```python
from build123d import *

# Parameters (mm, degrees)
SKETCH1_W           = 165
SKETCH1_H           = 50
BOSS_EXTRUDE1_DEPTH = 2.5
FILLET1_R           = 25
SKETCH2_R           = 2.5
CUT_EXTRUDE1_DEPTH  = 2.5
SKETCH4_R           = 2.25
BOSS_EXTRUDE2_DEPTH = 8


with BuildPart() as part:
    # Sketch1 → Boss-Extrude1 (new body)
    with BuildSketch(Plane.XY):
        Rectangle(SKETCH1_W, SKETCH1_H)
    extrude(amount=BOSS_EXTRUDE1_DEPTH)

    # Fillet1
    fillet1_edges = [part.edges().sort_by_distance(p)[0] for p in [
        (-82.5, -25, 1.25),
        (-82.5, 25, 1.25),
        (82.5, -25, 1.25),
        (82.5, 25, 1.25),
    ]]
    fillet(fillet1_edges, radius=FILLET1_R - 0.0001)  # a hair under: the kernel refuses the full size

    # Sketch2 → Cut-Extrude1 (cut)
    with BuildSketch(Plane.XY.offset(2.5)):
        with Locations((-5, 20)):
            Circle(SKETCH2_R)
        with Locations((5, 20)):
            Circle(SKETCH2_R)
    cut_extrude1 = extrude(amount=-CUT_EXTRUDE1_DEPTH, mode=Mode.SUBTRACT)

    # Mirror1: Cut-Extrude1 across plane
    add(cut_extrude1.mirror(Plane.ZX), mode=Mode.SUBTRACT)

    # Sketch4 → Boss-Extrude2 (add)
    with BuildSketch(Plane.XY.offset(2.5)):
        with Locations(Location((-57.5, 0, 0), (0, 0, 180))):
            Circle(SKETCH4_R)
    boss_extrude2 = extrude(amount=BOSS_EXTRUDE2_DEPTH)

    # Mirror3: Boss-Extrude2 across plane
    add(boss_extrude2.mirror(Plane(origin=(0, 0, 0), x_dir=(0, 0, 1), z_dir=(1, 0, 0))))


solid = part.part
```
Build history of the part. All positions in model axes, mm. A direction names the side the tool comes from. Give positions to 0.01 mm unless a question says otherwise; leave off trailing zeros. Loops run counter-clockwise (first coordinate to the right, second up) from the corner with the lowest first, then second, coordinate; pieces in that order, holes last. Notation, with made-up numbers: (20.5, 26.25) -> (30.5, 26.25) arc R15 cw to (30.5, 32.25) -> close; hole circle Ø3 at (-6.75, 13.25). An arc over 180 degrees is marked (long way). One line per question, with ' | ' between items. Start each with the question number.
1) Pin check, flat tips, straight feed: pin 1 (12 mm diameter, centred on x = 15.5, y = 17.5, fed in from +Z); pin 2 (3 mm diameter, centred on x = -5, y = -20, fed in from -Z); pin 3 (1 mm diameter, centred on y = -1, z = 5, fed in from +X). Stop position of each tip, or through.
2) Cut at C-C (x = 36.5). Give the cut face in (y, z), plus the area to 3 significant figures.
3) Cut at B-B (z = 4.25). Give the cut face in (x, y).
4) Probe L1, parallel to Y at x = -5, z = 1.4; L2, parallel to X at y = -20, z = 0.9; L3, parallel to Z at x = -32, y = -5. List the from-to ranges inside material, lowest first.
5) 3-axis set-ups, long thin cutter, end or side, ignore diameter. For faces 1 (the cylindrical face through (-3.66, -22.11, 1.27)), 2 (the cylindrical face through (55.252, -0.099, 6.444)): which of +Z, -Z, +X, -X, +Y, -Y reach the whole face in a straight line?
6) Two-plate mould, pull along X, no slides. Class faces 3 (the cylindrical face through (6.34, -22.11, 1.27)), 4 (the cylindrical face through (-75.371, 17.482, 1.268)), 5 (the cylindrical face through (74.982, -17.871, 1.268)): released by +X, released by -X, zero draft, split by the parting line, or undercut.
7) Cut at A-A (x = 5). Give the cut face in (y, z).
8) Cut at D-D (y = 13.5). Give the cut face in (x, z), plus the area to 3 significant figures.
Return value:
1) pin 1: z = 2.5 | pin 2: through | pin 3: x = 59.69
2) outline: (-25, 0) -> (25, 0) -> (25, 2.5) -> (-25, 2.5) -> close | area: 125 mm^2
3) outline: circle Ø4.5 at (-57.5, 0); circle Ø4.5 at (57.5, 0)
4) L1: -25 to -22.5, -17.5 to 17.5, 22.5 to 25 | L2: -72.5 to -7.5, -2.5 to 2.5, 7.5 to 72.5 | L3: 0 to 2.5
5) face 1: +Z, -Z | face 2: +Z
6) face 3: undercut | face 4: released by -X | face 5: released by +X
7) outline: (-25, 0) -> (-22.5, 0) -> (-22.5, 2.5) -> (-25, 2.5) -> close; (-17.5, 0) -> (17.5, 0) -> (17.5, 2.5) -> (-17.5, 2.5) -> close; (22.5, 0) -> (25, 0) -> (25, 2.5) -> (22.5, 2.5) -> close
8) outline: (-78.54, 0) -> (78.54, 0) -> (78.54, 2.5) -> (-78.54, 2.5) -> close | area: 393 mm^2
